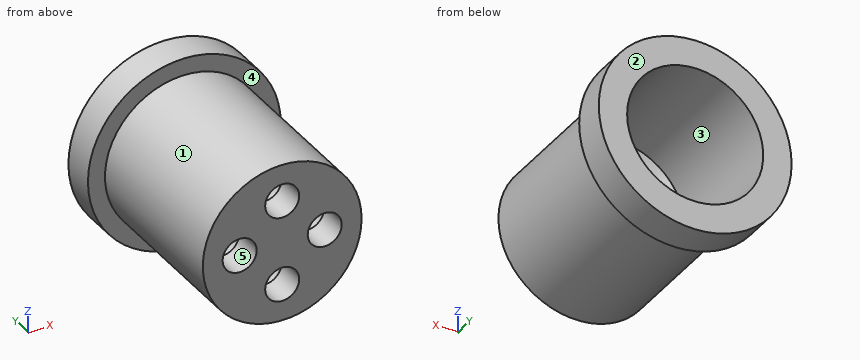
```python
from build123d import *

# Parameters (mm, degrees)
F0_R     = 8.5
F1_DEPTH = 3
F2_R     = 7
F3_DEPTH = 15
F5_D     = 3
F7_D     = 12
F7_DEPTH = 12
F7_TIP   = 3.6051637142
F9_D     = 4
F9_DEPTH = 15
F9_TIP   = 1.2017212381


with BuildPart() as f1:
    # F0 (on Front) → F1 (new body)
    with BuildSketch(Plane.XZ):
        Circle(F0_R)
    extrude(amount=F1_DEPTH)

    # F2 (on face) → F3 (join)
    with BuildSketch(Plane.XZ.offset(3)):
        Circle(F2_R)
    extrude(amount=F3_DEPTH)

    # F5 (through all)
    with Locations(Plane.XZ.offset(18)):
        with Locations((0, 3.75), (3.75, 0), (0, -3.75), (-3.75, 0)):
            Hole(F5_D / 2)

    # F7
    with Locations(Plane(origin=(0, 0, 0), x_dir=(-1, 0, 0), z_dir=(0, 1, 0))):
        with Locations((0, 0)):
            Hole(F7_D / 2, depth=F7_DEPTH)
            with Locations((0, 0, -(F7_DEPTH + F7_TIP / 2))):  # 118° drill point
                Cone(0, F7_D / 2, F7_TIP, mode=Mode.SUBTRACT)

    # F9
    with Locations(Plane(origin=(0, 0, 0), x_dir=(-1, 0, 0), z_dir=(0, 1, 0))):
        with Locations((0, 3.75), (-3.75, 0), (3.75, 0), (0, -3.75)):
            Hole(F9_D / 2, depth=F9_DEPTH)
            with Locations((0, 0, -(F9_DEPTH + F9_TIP / 2))):  # 118° drill point
                Cone(0, F9_D / 2, F9_TIP, mode=Mode.SUBTRACT)


solid = f1.part
```
Could you check a few things on this model? Use its own coordinates, in mm. Face numbers are marked on the shaded views. A direction names the side the tool comes from. Coordinates: 2 decimals unless noted, no trailing zeros. Order: outer loops, then holes, each group sorted by start corner. A loop starts at its lowest first (then second) coordinate and runs counter-clockwise, first axis right, second up. Notation, with made-up numbers: M 47,68.5 L 72,68.5 A35 cw 72,107.5 Z; hole C -32,0 d8. An arc over 180 degrees is marked long. Use a Markdown table: item, result. Add a question column.
Q1. Which directions (+Z, -Z, +X, -X, +Y, -Y) give clear straight access to the entire face, cutting with the end or side of a thin tool? Please do the marked faces 4 and 5.
Q2. I want a section at A-A on y = -12.5. List the corners of the cut face in (x, z) for me, then the cut area to 3 significant figures.
Q3. If I drill on L1, parallel to Z at x = 0, y = -16.2; L2, parallel to Z at x = 0, y = -5; L3, parallel to Y at x = -7, z = 1.75, over which ranges is the centre line in solid material (lowest first)?
Q4. I'm going to push flat-ended pins straight in: pin 1 (8 mm diameter, centred on y = -8.5, z = -4.5, fed in from +X); pin 2 (1.5 mm diameter, centred on x = 1, y = -10.5, fed in from +Z); pin 3 (5 mm diameter, centred on y = -3.5, z = -5.5, fed in from -X). Where does each tip first touch, or does it pass through?
Q5. I want a section at B-B on y = -16.25. List the corners of the cut face in (x, z) for me, then the cut area to 3 significant figures.
Q6. We'd pull the mould along Z, two halves only. Please class the marked faces 1, 2 and 3: pulls with the +Z half, pulls with the -Z half, needs draft (parallel to the pull), parting line crosses it, or undercut.
Q7. I want a section at D-D on x = -1.25. Give the number of separate pieces and of enclosed holes in the cut face, then the cut area to 3 significant figures.
Q8. I want a section at C-C on z = -7.5. List the corners of the cut face in (x, y) for me, then the cut area to 3 significant figures.
Checked values:
| question | item | result |
|---|---|---|
| 1 | face 4 | -Y |
| 1 | face 5 | +Y, -Y |
| 2 | outline | C 0,0 d14; hole M -4.9,-1.63 A5.17 ccw -1.63,-4.9 A2 ccw 1.63,-4.9 A5.17 ccw 4.9,-1.63 A2 ccw 4.9,1.63 A5.17 ccw 1.63,4.9 A2 ccw -1.63,4.9 A5.17 ccw -4.9,1.63 A2 ccw Z |
| 2 | area | 64.6 mm² |
| 3 | L1 | -7 to -5.25, -2.25 to 2.25, 5.25 to 7 |
| 3 | L2 | -7 to -6, 6 to 7 |
| 3 | L3 | -3 to 0 |
| 4 | pin 1 | x = 6.98 |
| 4 | pin 2 | z = 7 |
| 4 | pin 3 | x = -7.93 |
| 5 | outline | C 0,0 d14; hole C -3.75,0 d3; hole C 0,-3.75 d3; hole C 0,3.75 d3; hole C 3.75,0 d3 |
| 5 | area | 126 mm² |
| 6 | face 1 | parting line crosses it |
| 6 | face 2 | needs draft |
| 6 | face 3 | undercut |
| 7 | separate pieces | 3 |
| 7 | enclosed holes | 0 |
| 7 | area | 75.7 mm² |
| 8 | outline | M -4,-3 L 4,-3 L 4,0 L -4,0 Z |
| 8 | area | 24.0 mm² |
